Input: part model. Units: mm. Frame: model coordinates. A direction names the side the tool comes from. Coordinates: 2 decimals unless noted, no trailing zeros. Order: outer loops, then holes, each group sorted by start corner. A loop starts at its lowest first (then second) coordinate and runs counter-clockwise, first axis right, second up. Notation, with made-up numbers: M 30.25,-21.5 L 85.25,-21.5 A24 ccw 85.25,6.5 Z; hole C 3.25,87.25 d10. An arc over 180 degrees is marked long. Answer in a Markdown table with one row per item.
from build123d import *

# Parameters (mm, degrees)
SKETCH1_W           = 11.684
SKETCH1_H           = 33.02
BOSS_EXTRUDE1_DEPTH = 3.175
SKETCH2_W           = 11.684
SKETCH2_H           = 3.175
BOSS_EXTRUDE2_DEPTH = 12.7
CUT_EXTRUDE2_REACH  = 35.02
SKETCH3_R           = 1.778
FILLET2_R           = 2.54


with BuildPart() as part:
    # Sketch1 → Boss-Extrude1 (new body)
    with BuildSketch(Plane.XY):
        with Locations((0.021673222, 0)):
            Rectangle(SKETCH1_W, SKETCH1_H)
        with BuildLine():
            Line((-1.756326778, 5.588), (-1.756326778, 10.668))
            ThreePointArc((-1.756326778, 10.668), (0.021673222, 12.446), (1.799673222, 10.668))
            Line((1.799673222, 10.668), (1.799673222, 5.588))
            ThreePointArc((1.799673222, 5.588), (0.021673222, 3.81), (-1.756326778, 5.588))
        make_face(mode=Mode.SUBTRACT)
        with BuildLine():
            Line((-1.756326778, -5.588), (-1.756326778, -10.668))
            ThreePointArc((-1.756326778, -10.668), (0.021673222, -12.446), (1.799673222, -10.668))
            Line((1.799673222, -10.668), (1.799673222, -5.588))
            ThreePointArc((1.799673222, -5.588), (0.021673222, -3.81), (-1.756326778, -5.588))
        make_face(mode=Mode.SUBTRACT)
    extrude(amount=BOSS_EXTRUDE1_DEPTH)

    # Sketch2 → Boss-Extrude2 (add)
    with BuildSketch(Plane.XY.offset(3.175)):
        with Locations((0.021673222, 14.9225)):
            Rectangle(SKETCH2_W, SKETCH2_H)
    extrude(amount=BOSS_EXTRUDE2_DEPTH)

    # Sketch3 → Cut-Extrude2 (cut, up to next)
    with BuildSketch(Plane(origin=(0, 16.51, 0), x_dir=(1, 0, 0), z_dir=(0, 1, 0)), mode=Mode.PRIVATE) as cut_extrude2_sk1:
        with Locations((-2.899326778, -6.35)):
            Circle(SKETCH3_R)
    cut_extrude2_tool1 = extrude(cut_extrude2_sk1.sketch, amount=-CUT_EXTRUDE2_REACH, mode=Mode.PRIVATE) & part.part
    add(cut_extrude2_tool1.solids().sort_by_distance((-2.899327, 16.51, 6.35))[0], mode=Mode.SUBTRACT)
    # Sketch3 → Cut-Extrude2 (cut, up to next)
    with BuildSketch(Plane(origin=(0, 16.51, 0), x_dir=(1, 0, 0), z_dir=(0, 1, 0)), mode=Mode.PRIVATE) as cut_extrude2_sk2:
        with Locations((2.942673222, -6.35)):
            Circle(SKETCH3_R)
    cut_extrude2_tool2 = extrude(cut_extrude2_sk2.sketch, amount=-CUT_EXTRUDE2_REACH, mode=Mode.PRIVATE) & part.part
    add(cut_extrude2_tool2.solids().sort_by_distance((2.942673, 16.51, 6.35))[0], mode=Mode.SUBTRACT)
    # Sketch3 → Cut-Extrude2 (cut, up to next)
    with BuildSketch(Plane(origin=(0, 16.51, 0), x_dir=(1, 0, 0), z_dir=(0, 1, 0)), mode=Mode.PRIVATE) as cut_extrude2_sk3:
        with Locations((-2.899326778, -12.7)):
            Circle(SKETCH3_R)
    cut_extrude2_tool3 = extrude(cut_extrude2_sk3.sketch, amount=-CUT_EXTRUDE2_REACH, mode=Mode.PRIVATE) & part.part
    add(cut_extrude2_tool3.solids().sort_by_distance((-2.899327, 16.51, 12.7))[0], mode=Mode.SUBTRACT)
    # Sketch3 → Cut-Extrude2 (cut, up to next)
    with BuildSketch(Plane(origin=(0, 16.51, 0), x_dir=(1, 0, 0), z_dir=(0, 1, 0)), mode=Mode.PRIVATE) as cut_extrude2_sk4:
        with Locations((2.942673222, -12.7)):
            Circle(SKETCH3_R)
    cut_extrude2_tool4 = extrude(cut_extrude2_sk4.sketch, amount=-CUT_EXTRUDE2_REACH, mode=Mode.PRIVATE) & part.part
    add(cut_extrude2_tool4.solids().sort_by_distance((2.942673, 16.51, 12.7))[0], mode=Mode.SUBTRACT)

    # Fillet2
    fillet2_edges = [part.edges().sort_by_distance(p)[0] for p in [
        (-5.820326778, 14.9225, 15.875),
        (5.863673222, 14.9225, 15.875),
        (5.863673222, -16.51, 1.5875),
        (-5.820326778, -16.51, 1.5875),
    ]]
    fillet(fillet2_edges, radius=FILLET2_R)


solid = part.part
1) Mould query, pull axis Z, two halves, no side actions, for faces 1 (the face through (0, 13.335, 9)), 2 (the face through (-5.096, 14.945, 15.111)), 3 (the face through (-2.08, 14.94, 14.28)), 4 (the face through (0, 0, 0)). Classes: +Z half, -Z half, draft (parallel to the pull), parting line (faces both ways), or undercut.
Resolved:
| item | result |
|---|---|
| face 1 | draft |
| face 2 | +Z half |
| face 3 | undercut |
| face 4 | -Z half |
2) Material intervals for probe 1 along X at (y, z) = (15.3, 12.7); probe 2 along Z at (x, y) = (-4.75, 0.5) (3 decimals); probe 3 along Y at (x, z) = (1.75, 7.75) (3 decimals), sorted ascending.
Resolved:
| item | result |
|---|---|
| probe 1 | x = -5.82 to -4.68, -1.12 to 1.16, 4.72 to 5.86 |
| probe 2 | z = 0 to 3.175 |
| probe 3 | y = 13.335 to 16.51 |
3) Contact query for flat-ended pins moving along their axis: pin 1 (5 mm diameter, centred on y = 3.5, z = 8, fed in from +X) (3 decimals); pin 2 (1.5 mm diameter, centred on x = -3.5, z = 2, fed in from -Y); pin 3 (6 mm diameter, centred on x = 1.5, z = 7, fed in from -Y) (3 decimals); pin 4 (3.5 mm diameter, centred on x = 2.5, y = 5, fed in from +Z) (3 decimals). Output: stop coordinate, or through.
Resolved:
| item | result |
|---|---|
| pin 1 | passes through |
| pin 2 | stops at y = -16.51 |
| pin 3 | stops at y = 13.335 |
| pin 4 | stops at z = 3.175 |
4) Cut plane C-C, the plane x = 0. Output: boundary loops of the cut face in (y, z) (3 decimals).
Resolved:
| item | result |
|---|---|
| outline | M -16.51,0 L -12.446,0 L -12.446,3.175 L -16.51,3.175 Z; M -3.81,0 L 3.81,0 L 3.81,3.175 L -3.81,3.175 Z; M 12.446,0 L 16.51,0 L 16.51,15.875 L 13.335,15.875 L 13.335,3.175 L 12.446,3.175 Z |
5) Cut plane A-A, the plane z = 2. Output: boundary loops of the cut face in (x, y).
Resolved:
| item | result |
|---|---|
| outline | M -5.82,-13.97 A2.54 ccw -3.28,-16.51 L 3.32,-16.51 A2.54 ccw 5.86,-13.97 L 5.86,16.51 L -5.82,16.51 Z; hole M -1.76,-10.67 A1.78 ccw 1.8,-10.67 L 1.8,-5.59 A1.78 ccw -1.76,-5.59 Z; hole M -1.76,5.59 A1.78 ccw 1.8,5.59 L 1.8,10.67 A1.78 ccw -1.76,10.67 Z |
6) Cut plane D-D, the plane z = 6.35. Output: boundary loops of the cut face in (x, y) (3 decimals).
Resolved:
| item | result |
|---|---|
| outline | M -5.82,13.335 L -4.677,13.335 L -4.677,16.51 L -5.82,16.51 Z; M -1.121,13.335 L 1.165,13.335 L 1.165,16.51 L -1.121,16.51 Z; M 4.721,13.335 L 5.864,13.335 L 5.864,16.51 L 4.721,16.51 Z |
7) Cut plane B-B, the plane y = -6.5. Output: boundary loops of the cut face in (x, z) (3 decimals), and give its area (3 significant figures).
Resolved:
| item | result |
|---|---|
| outline | M -5.82,0 L -1.756,0 L -1.756,3.175 L -5.82,3.175 Z; M 1.8,0 L 5.864,0 L 5.864,3.175 L 1.8,3.175 Z |
| area | 25.8 mm2 |
8) Reachability of faces 5 (the face through (0, -1, 3.175)), 6 (the face through (1.8, -8, 2)), 7 (the face through (-5.82, 6, 2)) from +Z, -Z, +X, -X, +Y, -Y: full face, straight path, thin tool, end or side. Return the list, or none.
Resolved:
| item | result |
|---|---|
| face 5 | +Z, +X, -X, -Y |
| face 6 | +Z, -Z |
| face 7 | +Z, -Z, -X, +Y, -Y |
